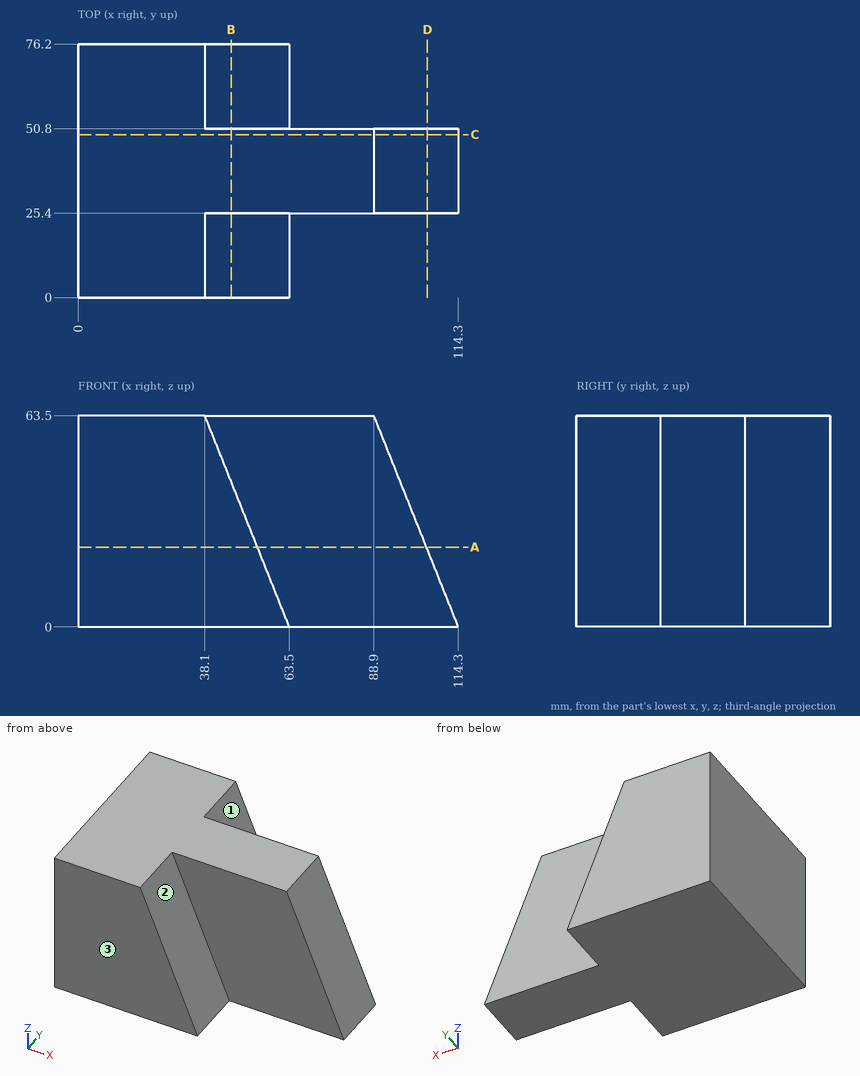
Geometry: see drawing. Coordinates: mm, zero at the bounding-box minimum. A direction names the side the tool comes from. Coordinates: 2 decimals unless noted, no trailing zeros. Order: outer loops, then holes, each group sorted by start corner. A loop starts at its lowest first (then second) coordinate and runs counter-clockwise, first axis right, second up. Notation, with made-up numbers: M 69,38 L 95,38 A27 cw 95,63 Z; hole C 60.5,85 d3. An arc over 180 degrees is marked long. Answer in a Markdown table with one row per item. Add a question column.
Q1. Contact query for flat-ended pins moving along their axis: P1, Ø12, axis at y = 45, z = 57, coming from the +X side; P2, Ø5, axis at y = 59, z = 43, coming from the +X side; P3, Ø1, axis at x = 81, z = 38.5, coming from the -Y side. Output: stop coordinate, or through.
Q2. Section query D-D on x = 105. Return the cut outline in (y, z).
Q3. Reachability of the marked faces 1, 2 and 3 from +Z, -Z, +X, -X, +Y, -Y: full face, straight path, thin tool, end or side. Return the list, or none.
Q4. Section query B-B on x = 46. Return the cut outline in (y, z).
Q5. Line query: L1, parallel to Y at x = 76.5, z = 56.5; L2, parallel to X at y = 12.5, z = 39; L3, parallel to X at y = 71, z = 34. Output: solid intervals per line, ascending.
Q6. Section query A-A on z = 24. Return the cut outline in (x, y).
Q7. Section query C-C on y = 49. Return the cut outline in (x, z).
Completed:
| question | item | result |
|---|---|---|
| 1 | P1 | stops at x = 93.9 |
| 1 | P2 | stops at x = 47.3 |
| 1 | P3 | stops at y = 25.4 |
| 2 | outline | M 25.4,0 L 50.8,0 L 50.8,23.25 L 25.4,23.25 Z |
| 3 | face 1 | +Z, +X, +Y |
| 3 | face 2 | +Z, +X, -Y |
| 3 | face 3 | +Z, -Z, +X, -X, -Y |
| 4 | outline | M 0,0 L 76.2,0 L 76.2,43.75 L 50.8,43.75 L 50.8,63.5 L 25.4,63.5 L 25.4,43.75 L 0,43.75 Z |
| 5 | L1 | y = 25.4 to 50.8 |
| 5 | L2 | x = 0 to 47.9 |
| 5 | L3 | x = 0 to 49.9 |
| 6 | outline | M 0,0 L 53.9,0 L 53.9,25.4 L 104.7,25.4 L 104.7,50.8 L 53.9,50.8 L 53.9,76.2 L 0,76.2 Z |
| 7 | outline | M 0,0 L 114.3,0 L 88.9,63.5 L 0,63.5 Z |
